```python
from build123d import *

# Parameters (mm, degrees)
BOX_W       = 76.2
BOX_H       = 1590.55
BOX_DEPTH   = 76.2
THICKNESS_T = -3.175


with BuildPart() as part:
    # Box → Box (new body)
    with BuildSketch(Plane.XY):
        with Locations((38.1, 795.275)):
            Rectangle(BOX_W, BOX_H)
    extrude(amount=BOX_DEPTH)

    # Thickness
    thickness_openings = [part.faces().sort_by_distance(p)[0] for p in [
        (38.1, 0, 38.1),
        (38.1, 1590.55, 38.1),
    ]]
    offset(amount=THICKNESS_T, openings=thickness_openings)


solid = part.part
```
The model under review builds one solid part; all positions refer to its coordinate system, in mm. A direction names the side the tool comes from. Round coordinates to 2 decimals unless told otherwise and drop trailing zeros. Write each loop counter-clockwise with the first axis right and the second up, starting at its lowest first coordinate (ties: lowest second). Pieces come first, ordered by that corner, then holes. Notation, with made-up numbers: (30, -33.5) - (68, -33.5) arc R23 ccw to (68, -4.5) - close; hole circle Ø11 at (54.25, 79). An arc over 180 degrees is marked (long way). Answer as CSV lines item,"result". Start each with the question number.
(1) We need section C-C on y = 296.5. State the section outline as (x, z) points (3 decimals), plus the area to 3 significant figures.
(2) We need section A-A on z = 41.5. State the section outline as (x, y) points (3 decimals), plus the area to 3 significant figures.
(3) We need section B-B on x = 15.5. State the section outline as (y, z) points (3 decimals), plus the area to 3 significant figures.
(4) To check wall thickness, follow line 1 (X direction, y = 889, z = 10) (3 decimals). State the ranges of the line that lie inside material, in increasing order.
(5) For faces 1 (the flat face through (38, 806, 3.175)), 2 (the flat face through (35, 1590.55, 75)), list the 3-axis set-ups (+Z, -Z, +X, -X, +Y, -Y) from which the entire face can be reached by the end or side of a thin tool; tool diameter is ignored.
(6) Draft analysis for pull direction Z (two halves, no side actions). For faces 3 (the flat face through (73.025, 784, 38)), 4 (the flat face through (38, 806, 0)), 5 (the flat face through (76.2, 784, 38)), state which applies: pulls with the +Z half, pulls with the -Z half, needs draft (parallel to the pull), parting line crosses it, or undercut.
(7) For pin 1 Ø8 at (x, y) = (30, 1093) entering from -Z, flat-tipped, find the tip position at first contact; note if it passes through.
Worked answers:
1,outline,"(0, 0) - (76.2, 0) - (76.2, 76.2) - (0, 76.2) - close; hole (3.175, 3.175) - (73.025, 3.175) - (73.025, 73.025) - (3.175, 73.025) - close"
1,area,"927 mm²"
2,outline,"(0, 0) - (3.175, 0) - (3.175, 1590.55) - (0, 1590.55) - close; (73.025, 0) - (76.2, 0) - (76.2, 1590.55) - (73.025, 1590.55) - close"
2,area,"10,100 mm²"
3,outline,"(0, 0) - (1590.55, 0) - (1590.55, 3.175) - (0, 3.175) - close; (0, 73.025) - (1590.55, 73.025) - (1590.55, 76.2) - (0, 76.2) - close"
3,area,"10,100 mm²"
4,line 1,"0 to 3.175, 73.025 to 76.2"
5,face 1,"+Y, -Y"
5,face 2,"+Z, -Z, +X, -X, +Y"
6,face 3,"undercut"
6,face 4,"pulls with the -Z half"
6,face 5,"needs draft"
7,pin 1,"z = 0"
